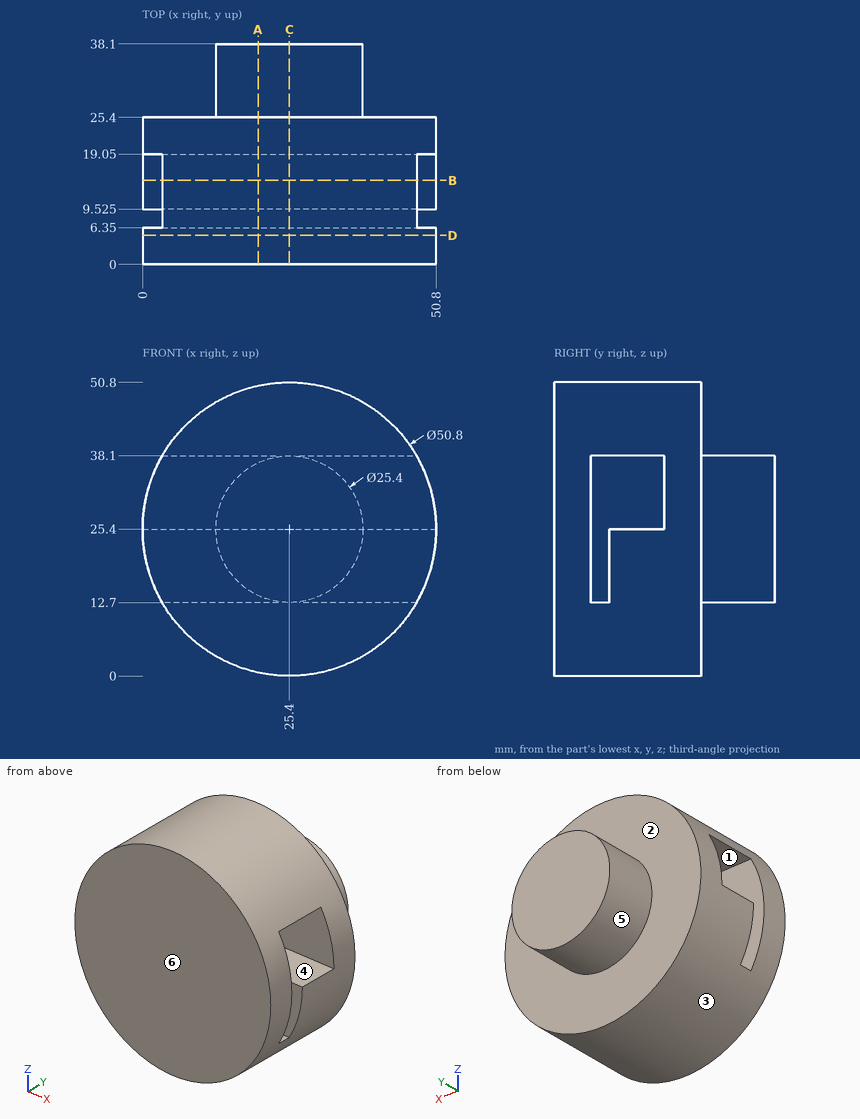
Answer from the drawing. Dimensions are ordinates in mm from the lowest x, y and z of the part. A direction names the side the tool comes from. Coordinates: 2 decimals unless noted, no trailing zeros. Write each loop counter-clockwise with the first axis right and the second up, starting at its lowest first coordinate (ties: lowest second). Pieces come first, ordered by that corner, then holes. Notation, with made-up numbers: (28.5, 26) -> (69.5, 26) arc R36 ccw to (69.5, 64) -> close; hole circle Ø6 at (38, 58.25). An arc over 180 degrees is marked (long way). One line per question, with ' | ' between items.
1. Section B-B (y = 14.5) is taken. Determine the outline of the cut face in (x, z), and give its area (3 significant figures).
Verdict:
outline: (0, 25.4) arc R25.4 ccw to (50.8, 25.4) -> close; (3.4, 38.1) -> (47.4, 38.1) arc R25.4 ccw to start | area: 1,410 mm^2
2. Section A-A (x = 20) is taken. Determine the outline of the cut face in (y, z) (3 decimals).
Verdict:
outline: (0, 0.581) -> (25.4, 0.581) -> (25.4, 13.905) -> (38.1, 13.905) -> (38.1, 36.895) -> (25.4, 36.895) -> (25.4, 50.219) -> (0, 50.219) -> close; hole (6.35, 12.7) -> (9.525, 12.7) -> (9.525, 25.4) -> (19.05, 25.4) -> (19.05, 38.1) -> (6.35, 38.1) -> close
3. Section D-D (y = 5) is taken. Determine the outline of the cut face in (x, z), and give its area (3 significant figures).
Verdict:
outline: circle Ø50.8 at (25.4, 25.4) | area: 2,030 mm^2
4. Given pin 1 Ø3 at (x, y) = (22.5, 16.5) entering from +Z; pin 2 Ø8 at (y, z) = (6, 37.5) entering from -X; pin 3 Ø10 at (x, z) = (28.5, 18) entering from -Y; pin 4 Ø3 at (x, y) = (39, 22.5) entering from +Z, each flat-ended and moving along its own axis, determine where each tip first touches the part or whether it passes through.
Verdict:
pin 1: stops at z = 50.76 | pin 2: stops at x = 1.33 | pin 3: stops at y = 0 | pin 4: stops at z = 47.73
5. Straight lines are drawn through the part: line 1 (Y direction, x = 38, z = 21) (3 decimals); line 2 (Y direction, x = 9, z = 26.5); line 3 (Y direction, x = 38, z = 5). For each, find the intervals that lie inside material, in ascending order.
Verdict:
line 1: y = 0 to 6.35, 9.525 to 25.4 | line 2: y = 0 to 6.35, 19.05 to 25.4 | line 3: y = 0 to 25.4
6. Section C-C (x = 25.4) is taken. Determine the outline of the cut face in (y, z) (3 decimals), and give its area (3 significant figures).
Verdict:
outline: (0, 0) -> (25.4, 0) -> (25.4, 12.7) -> (38.1, 12.7) -> (38.1, 38.1) -> (25.4, 38.1) -> (25.4, 50.8) -> (0, 50.8) -> close; hole (6.35, 12.7) -> (9.525, 12.7) -> (9.525, 25.4) -> (19.05, 25.4) -> (19.05, 38.1) -> (6.35, 38.1) -> close | area: 1,410 mm^2
7. For a pull along Z with two mould halves and no side action, classify the marked faces 4, 5 and 6 as released by +Z, released by -Z, zero draft, split by the parting line, or undercut.
Verdict:
face 4: undercut | face 5: split by the parting line | face 6: zero draft
8. Which of the six approach directions +Z, -Z, +X, -X, +Y, -Y give full straight-line access (tool end or side, diameter ignored) to the marked faces 1, 2 and 3?
Verdict:
face 1: +X, -X | face 2: +Y | face 3: +Y, -Y
